Here's how the part is built. I have some questions about the finished solid (model axes, mm). A direction names the side the tool comes from. Round coordinates to 2 decimals unless told otherwise and drop trailing zeros. Loops run counter-clockwise (first coordinate to the right, second up) from the corner with the lowest first, then second, coordinate; pieces in that order, holes last. Notation, with made-up numbers: M 29,50 L 39,50 A21 ccw 39,70 Z; hole C 31,18 d9. An arc over 180 degrees is marked long. Answer as CSV lines item,"result".
```python
from build123d import *

# Parameters (mm, degrees)
SKETCH2_W                                      = 100.5
SKETCH2_H                                      = 166.5
SKETCH2_W_2                                    = 98.5
SKETCH2_H_2                                    = 164.5
DIAPLAY_RING_DEPTH                             = 3.5
SKETCH3_W                                      = 100.5
SKETCH3_H                                      = 166.5
SKETCH3_W_2                                    = 92.5
SKETCH3_H_2                                    = 158.5
DISPLAY_LIP_DEPTH                              = 2
SKETCH4_W                                      = 16
SKETCH4_H                                      = 12
SKETCH4_R                                      = 1.75
DISPLAY_MOUNTING_TABS_DEPTH                    = 8
FILLET1_R                                      = 6
SKETCH7_W                                      = 100.5
SKETCH7_H                                      = 166.5
SKETCH7_W_2                                    = 96.5
SKETCH7_H_2                                    = 162.5
PERIMETER_EXTENSION_FOR_STRUCTURE_DEPTH        = 7
PERIMETER_EXTENSION_FOR_CAR_TRIM_DEPTH         = 2
SKETCH9_W                                      = 4
SKETCH9_H                                      = 166.5
MATERIAL_ADDITION_FOR_DISPLAY_MOUNTING_S_DEPTH = 4
SKETCH10_W                                     = 150
SKETCH10_H                                     = 1.25
DISPLAY_MOUNTING_SLOT_DEPTH                    = 3
SKETCH6_R                                      = 1.75
SHIFTER_SCREW_IF_DEPTH                         = 3
CUT_EXTRUDE2_DEPTH                             = 137.888640873
CUT_EXTRUDE2_DEPTH_BACK                        = 137.888640873


with BuildPart() as part:
    # Sketch2 → DIAPLAY RING (new body)
    with BuildSketch(Plane(origin=(0, 0, 0), x_dir=(1, 0, 0), z_dir=(0, 1, 0))):
        Rectangle(SKETCH2_W, SKETCH2_H)
        Rectangle(SKETCH2_W_2, SKETCH2_H_2, mode=Mode.SUBTRACT)
    extrude(amount=DIAPLAY_RING_DEPTH)

    # Sketch3 → DISPLAY LIP (add)
    with BuildSketch(Plane(origin=(0, 0, 0), x_dir=(1, 0, 0), z_dir=(0, 1, 0))):
        Rectangle(SKETCH3_W, SKETCH3_H)
        Rectangle(SKETCH3_W_2, SKETCH3_H_2, mode=Mode.SUBTRACT)
    extrude(amount=-DISPLAY_LIP_DEPTH)

    # Sketch4 → DISPLAY MOUNTING TABS (add)
    # profile 1 of 2: a face of its own
    with BuildSketch(Plane(origin=(0, 0, 0), x_dir=(1, 0, 0), z_dir=(0, 1, 0))):
        with Locations((-42.25, -63.25)):
            Rectangle(SKETCH4_W, SKETCH4_H)
        with Locations(Location((-40.25, -63.25, 0), (0, 0, 270))):
            Circle(SKETCH4_R, mode=Mode.SUBTRACT)
    # profile 2 of 2: a face of its own
    with BuildSketch(Plane(origin=(0, 0, 0), x_dir=(1, 0, 0), z_dir=(0, 1, 0))):
        with Locations((-42.25, 36.75)):
            Rectangle(SKETCH4_W, SKETCH4_H)
        with Locations(Location((-40.25, 36.75, 0), (0, 0, 270))):
            Circle(SKETCH4_R, mode=Mode.SUBTRACT)
    extrude(amount=-DISPLAY_MOUNTING_TABS_DEPTH)

    # Fillet1
    fillet1_edges = [part.edges().sort_by_distance(p)[0] for p in [
        (-34.25, -4, 57.25),
        (-34.25, -4, 69.25),
        (-34.25, -4, -42.75),
        (-34.25, -4, -30.75),
    ]]
    fillet(fillet1_edges, radius=FILLET1_R - 0.0001)  # a hair under: the kernel refuses the full size

    # Sketch7 → PERIMETER EXTENSION FOR STRUCTURE (add)
    with BuildSketch(Plane(origin=(0, -1, 0), x_dir=(1, 0, 0), z_dir=(0, 1, 0))):
        Rectangle(SKETCH7_W, SKETCH7_H)
        Rectangle(SKETCH7_W_2, SKETCH7_H_2, mode=Mode.SUBTRACT)
    extrude(amount=-PERIMETER_EXTENSION_FOR_STRUCTURE_DEPTH)

    # Sketch8 → PERIMETER EXTENSION FOR CAR TRIM (add)
    with BuildSketch(Plane.XZ.offset(8)):
        Polygon((25.25, 83.25), (50.25, 83.25), (50.25, -83.25), (25.25, -83.25), (25.25, -81.25), (48.25, -81.25), (48.25, 81.25), (25.25, 81.25), align=None)
    extrude(amount=PERIMETER_EXTENSION_FOR_CAR_TRIM_DEPTH)

    # Sketch9 → MATERIAL ADDITION FOR DISPLAY MOUNTING SLOT (add)
    with BuildSketch(Plane(origin=(0, -1, 0), x_dir=(1, 0, 0), z_dir=(0, 1, 0))):
        with Locations((48.25, 0)):
            Rectangle(SKETCH9_W, SKETCH9_H)
    extrude(amount=-MATERIAL_ADDITION_FOR_DISPLAY_MOUNTING_S_DEPTH)

    # Sketch10 → DISPLAY MOUNTING SLOT (cut)
    with BuildSketch(Plane.ZY.offset(-46.25)):
        with Locations((0, -2.5)):
            Rectangle(SKETCH10_W, SKETCH10_H)
    extrude(amount=-DISPLAY_MOUNTING_SLOT_DEPTH, mode=Mode.SUBTRACT)

    # Sketch11 → Cut-Extrude2 (cut, two sides: drawn at the far end of the back side and taken through both)
    with BuildSketch(Plane.XY.offset(-CUT_EXTRUDE2_DEPTH_BACK)):
        Polygon((50.25, -10), (50.25, -5), (46.25, -5), (46.25, -2), (20.25, -2), (20.25, -10), align=None)
    extrude(amount=CUT_EXTRUDE2_DEPTH + CUT_EXTRUDE2_DEPTH_BACK, mode=Mode.SUBTRACT)


with BuildPart() as body_2:
    # Sketch6 → SHIFTER SCREW IF (new body)
    with BuildSketch(Plane(origin=(0, -55, 0), x_dir=(1, 0, 0), z_dir=(0, 1, 0))):
        with BuildLine():
            Line((-50, 106.5), (12, 106.5))
            ThreePointArc((12, 106.5), (25.5, 93), (12, 79.5))
            Line((12, 79.5), (-50, 79.5))
            ThreePointArc((-50, 79.5), (-63.5, 93), (-50, 106.5))
        make_face()
        with Locations(Location((-50, 93, 0), (0, 0, 270))):
            Circle(SKETCH6_R, mode=Mode.SUBTRACT)
        with Locations(Location((12, 93, 0), (0, 0, 270))):
            Circle(SKETCH6_R, mode=Mode.SUBTRACT)
    extrude(amount=-SHIFTER_SCREW_IF_DEPTH)


solid = part.part
```
1. I want a section at A-A, the plane x = -2. Please give me the cut outline in (y, z), and give its area (3 significant figures).
Evaluation:
outline,"M -8,-83.25 L 3.5,-83.25 L 3.5,-82.25 L 0,-82.25 L 0,-79.25 L -2,-79.25 L -2,-81.25 L -8,-81.25 Z; M -8,81.25 L -2,81.25 L -2,79.25 L 0,79.25 L 0,82.25 L 3.5,82.25 L 3.5,83.25 L -8,83.25 Z"
area,"47.0 mm²"
2. Which directions (+Z, -Z, +X, -X, +Y, -Y) give clear straight access to the entire face, cutting with the end or side of a thin tool? Please do faces 1 (the flat face through (48, -1.875, -1)), 2 (the flat face through (-44, -4, -42.75)), 3 (the flat face through (-37, 0, -37)).
Evaluation:
face 1,"none"
face 2,"-Y"
face 3,"+Y"
3. I want a section at B-B, the plane z = -63.5. Please give me the cut outline in (x, y) (3 decimals).
Evaluation:
outline,"M -50.25,-8 L -48.25,-8 L -48.25,-2 L -46.25,-2 L -46.25,0 L -49.25,0 L -49.25,3.5 L -50.25,3.5 Z; M 46.25,-5 L 50.25,-5 L 50.25,3.5 L 49.25,3.5 L 49.25,0 L 46.25,0 L 46.25,-1.875 L 49.25,-1.875 L 49.25,-3.125 L 46.25,-3.125 Z"
4. We'd pull the mould along X, two halves only. Please class faces 4 (the flat face through (48, -3.125, -1)), 5 (the flat face through (48, -5, -1)): pulls with the +X half, pulls with the -X half, needs draft (parallel to the pull), parting line crosses it, or undercut.
Evaluation:
face 4,"undercut"
face 5,"needs draft"
5. If I drill on line 1 (X direction, y = -4.5, z = 74); line 2 (Z direction, x = -40.5, y = -2.5); line 3 (X direction, y = 1.25, z = -11.5), over which ranges is the centre line in solid material (lowest first)? Write a range as [from, to].
Evaluation:
line 1,"x = [-50.25, -48.25], [46.25, 50.25]"
line 2,"z = [-83.25, -81.25], [-42.75, -38.48], [-35.02, -30.75], [57.25, 61.52], [64.98, 69.25], [81.25, 83.25]"
line 3,"x = [-50.25, -49.25], [49.25, 50.25]"
6. For P1, Ø0.9, axis at x = 48, z = -16, coming from the +Y side; P2, Ø3, axis at x = 49, z = 2, coming from the -Y side; P3, Ø4, axis at x = -11.5, z = 75.5, coming from the -Y side, each with a flat end and sliding along its axis, tell me the tip position at first contact or that it passes through.
Evaluation:
P1,"stops at y = 0"
P2,"stops at y = -5"
P3,"passes through"
